Source: CAD feature listing. Evaluate the final solid. Frame: model axes, mm. Face numbers are marked on the shaded views. A direction names the side the tool comes from. Coordinates: 2 decimals unless noted, no trailing zeros. Order: outer loops, then holes, each group sorted by start corner. A loop starts at its lowest first (then second) coordinate and runs counter-clockwise, first axis right, second up. Notation, with made-up numbers: (-20.75, 54) -> (1.25, 54) arc R30 ccw to (1.25, 87) -> close; hole circle Ø8 at (14.25, 14.25). An arc over 180 degrees is marked (long way). Put each result on its own line as item: value.
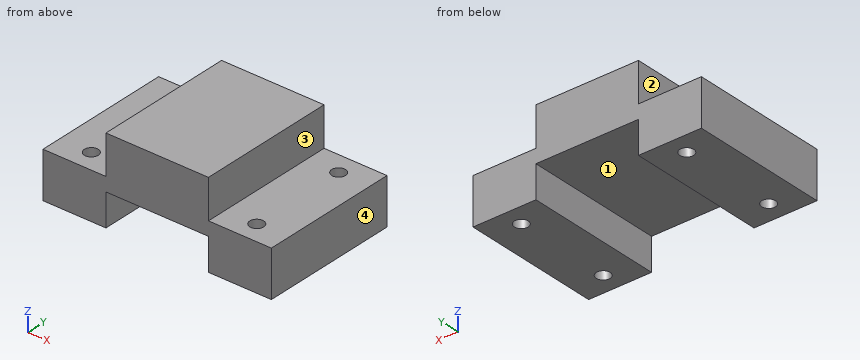
from build123d import *

# Parameters (mm, degrees)
F1_DEPTH = 76.2
F3_D     = 7.62
F5_D     = 7.62


with BuildPart() as f1:
    # F0 (on Front) → F1 (new body)
    with BuildSketch(Plane.XZ):
        Polygon((-62.504791, 0), (-28.054785, 0), (-28.054785, 17.78), (28.054785, 17.78), (28.054785, 0), (62.504791, 0), (62.504791, 25.4), (28.054785, 25.4), (28.054785, 46.863), (0, 46.863), (-28.054785, 46.863), (-28.054785, 25.4), (-62.504791, 25.4), align=None)
    extrude(amount=F1_DEPTH)

    # F3 (through all)
    with Locations(Plane.XY.offset(25.4)):
        with Locations((-45.279788, -11.107678), (-45.279788, -65.092322)):
            Hole(F3_D / 2)

    # F5 (through all)
    with Locations(Plane.XY.offset(25.4)):
        with Locations((45.279788, -11.107678), (45.279788, -65.092322)):
            Hole(F5_D / 2)


solid = f1.part
1. Set-up query: the marked faces 1, 2, 3 and 4. Return all of +Z, -Z, +X, -X, +Y, -Y with unobstructed straight access to the full face (end or side cutting, diameter ignored); none if empty.
Numbers:
face 1: -Z, +Y, -Y
face 2: +Z, -X, +Y, -Y
face 3: +Z, +X, +Y, -Y
face 4: +Z, -Z, +X, +Y, -Y
2. Cut plane B-B on y = -66.5. Output: boundary loops of the cut face in (x, z).
Numbers:
outline: (-62.5, 0) -> (-48.82, 0) -> (-48.82, 25.4) -> (-62.5, 25.4) -> close; (-41.74, 0) -> (-28.05, 0) -> (-28.05, 17.78) -> (28.05, 17.78) -> (28.05, 0) -> (41.74, 0) -> (41.74, 25.4) -> (28.05, 25.4) -> (28.05, 46.86) -> (-28.05, 46.86) -> (-28.05, 25.4) -> (-41.74, 25.4) -> close; (48.82, 0) -> (62.5, 0) -> (62.5, 25.4) -> (48.82, 25.4) -> close
3. Cut plane A-A on z = 14. Output: boundary loops of the cut face in (x, y).
Numbers:
outline: (-62.5, -76.2) -> (-28.05, -76.2) -> (-28.05, 0) -> (-62.5, 0) -> close; (28.05, -76.2) -> (62.5, -76.2) -> (62.5, 0) -> (28.05, 0) -> close; hole circle Ø7.62 at (-45.28, -65.09); hole circle Ø7.62 at (-45.28, -11.11); hole circle Ø7.62 at (45.28, -65.09); hole circle Ø7.62 at (45.28, -11.11)
4. First-contact query: pin 1 (9 mm diameter, centred on x = -45.28, y = -65.09, fed in from +Z); pin 2 (3 mm diameter, centred on x = -9.5, y = -38, fed in from -Z); pin 3 (10.5 mm diameter, centred on y = -23, z = 33.5, fed in from +X). Flat tips, straight axial feed; report the tip coordinate or a pass-through.
Numbers:
pin 1: stops at z = 25.4
pin 2: stops at z = 17.78
pin 3: stops at x = 28.05
5. Ray query, line 1 along X through (y, z) = (-22, 9.5); line 2 along X through (y, z) = (-67, 43.5); line 3 along Z through (x, y) = (14, -27.5). Return the intervals inside material, ascending.
Numbers:
line 1: x = -62.5 to -28.05, 28.05 to 62.5
line 2: x = -28.05 to 28.05
line 3: z = 17.78 to 46.86
6. Cut plane D-D on y = -40. Output: boundary loops of the cut face in (x, z).
Numbers:
outline: (-62.5, 0) -> (-28.05, 0) -> (-28.05, 17.78) -> (28.05, 17.78) -> (28.05, 0) -> (62.5, 0) -> (62.5, 25.4) -> (28.05, 25.4) -> (28.05, 46.86) -> (-28.05, 46.86) -> (-28.05, 25.4) -> (-62.5, 25.4) -> close
7. Cut plane C-C on x = 45. Output: boundary loops of the cut face in (y, z), plus the area to 3 significant figures.
Numbers:
outline: (-76.2, 0) -> (-68.89, 0) -> (-68.89, 25.4) -> (-76.2, 25.4) -> close; (-61.29, 0) -> (-14.91, 0) -> (-14.91, 25.4) -> (-61.29, 25.4) -> close; (-7.31, 0) -> (0, 0) -> (0, 25.4) -> (-7.31, 25.4) -> close
area: 1,550 mm2
